Answer from the drawing. Dimensions are ordinates in mm from the lowest x, y and z of the part. A direction names the side the tool comes from. Give positions to 0.01 mm unless a question says otherwise; leave off trailing zeros. Loops run counter-clockwise (first coordinate to the right, second up) from the corner with the lowest first, then second, coordinate; pieces in that order, holes last.
(1) Straight lines are drawn through the part: probe 1 along Z at (x, y) = (42, 3.2); probe 2 along Z at (x, y) = (8, 1.5); probe 3 along X at (y, z) = (10.75, 8). For each, find the intervals that lie inside material, in ascending order.
(2) Find section C-C, the plane x = 3. Write down the section's boundary in (y, z).
(3) Find section A-A, the plane x = 42. Write down the section's boundary in (y, z), then the cut area to 3 significant figures.
(4) Find section D-D, the plane z = 20.75. Write down the section's boundary in (x, y).
(5) Each of these flat-tipped pins is pushed along its axis until it touches: P1, Ø1.8, axis at x = 2.5, z = 13, coming from the +Y side; P2, Ø10, axis at y = 20, z = 11, coming from the +X side; P3, Ø10, axis at x = 36.5, z = 13, coming from the +Y side. Where does it stop, or does it pass through?
(6) Determine the mould class of the marked faces 1, 2 and 3 for opening direction X: pulls with the +X half, pulls with the -X half, needs draft (parallel to the pull), parting line crosses it, or undercut.
(7) Find section B-B, the plane y = 2. Write down the section's boundary in (x, z).
(8) Which of the six approach directions +Z, -Z, +X, -X, +Y, -Y give full straight-line access (tool end or side, diameter ignored) to the marked faces 4, 5, 6 and 7?
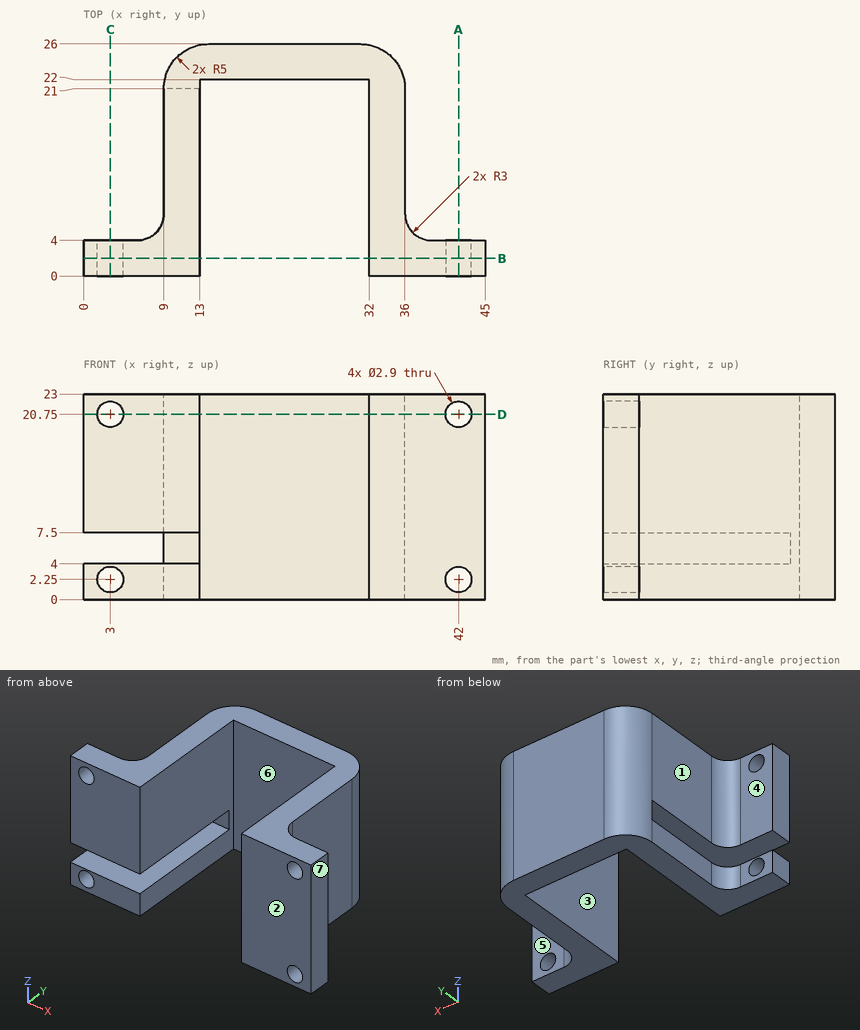
Entries:
1. probe 1: z = 0 to 0.8, 3.7 to 19.3, 22.2 to 23
1. probe 2: z = 0 to 4, 7.5 to 23
1. probe 3: x = 9 to 13, 32 to 36
2. outline: (0, 0) - (4, 0) - (4, 0.8) - (0, 0.8) - close; (0, 3.7) - (4, 3.7) - (4, 4) - (0, 4) - close; (0, 7.5) - (4, 7.5) - (4, 19.3) - (0, 19.3) - close; (0, 22.2) - (4, 22.2) - (4, 23) - (0, 23) - close
3. outline: (0, 0) - (4, 0) - (4, 0.8) - (0, 0.8) - close; (0, 3.7) - (4, 3.7) - (4, 19.3) - (0, 19.3) - close; (0, 22.2) - (4, 22.2) - (4, 23) - (0, 23) - close
3. area: 68.8 mm2
4. outline: (0, 0) - (1.55, 0) - (1.55, 4) - (0, 4) - close; (4.45, 0) - (13, 0) - (13, 22) - (32, 22) - (32, 0) - (40.55, 0) - (40.55, 4) - (39, 4) arc R3 cw to (36, 7) - (36, 21) arc R5 ccw to (31, 26) - (14, 26) arc R5 ccw to (9, 21) - (9, 7) arc R3 cw to (6, 4) - (4.45, 4) - close; (43.45, 0) - (45, 0) - (45, 4) - (43.45, 4) - close
5. P1: stops at y = 4
5. P2: stops at x = 36
5. P3: stops at y = 25.97
6. face 1: pulls with the -X half
6. face 2: needs draft
6. face 3: undercut
7. outline: (0, 0) - (13, 0) - (13, 4) - (0, 4) - close; (0, 7.5) - (13, 7.5) - (13, 23) - (0, 23) - close; (32, 0) - (45, 0) - (45, 23) - (32, 23) - close; hole circle Ø2.9 at (3, 2.25); hole circle Ø2.9 at (3, 20.75); hole circle Ø2.9 at (42, 2.25); hole circle Ø2.9 at (42, 20.75)
8. face 4: +Z, -Z, -X, +Y
8. face 5: +Z, -Z, +X, +Y
8. face 6: +Z, -Z, -Y
8. face 7: +Z, -Z, +X, +Y, -Y
